Part model, mm, in its own coordinate system. A direction names the side the tool comes from. Round coordinates to 2 decimals unless told otherwise and drop trailing zeros. Loops run counter-clockwise (first coordinate to the right, second up) from the corner with the lowest first, then second, coordinate; pieces in that order, holes last. Notation, with made-up numbers: M -1.75,-11.5 L 57.25,-11.5 A19 cw 57.25,-7.5 Z; hole C 29,48 d9. An arc over 180 degrees is marked long. Answer as CSV lines item,"result". Start each with the question number.
Item 1: Band-saw the part on B-B (z = -5.5). Give the cut face in (x, y).
Item 2: Mould opens along Z. For faces 1 (the flat face through (123, 1.5, 0)), 2 (the flat face through (249, 1, 0)), 3 (the flat face through (123, 8, 20)) say: pulls with the +Z half, pulls with the -Z half, needs draft (parallel to the pull), parting line crosses it, or undercut.
Item 3: Which spindle directions (+Z, -Z, +X, -X, +Y, -Y) get a long thin tool onto all of the face, cutting with end or side? Do faces 4 (the flat face through (123, 8, -18.5)), 5 (the flat face through (123, 0, 0)). Say none if no direction does.
Item 4: Band-saw the part on A-A (x = 60.5). Give the cut face in (y, z), and give its area (4 significant figures).
Item 5: Drop flat-ended pins along their axis: pin 1 Ø2 at (x, y) = (91.67, 7.5) entering from +Z; pin 2 Ø11 at (x, z) = (143, 5) entering from +Y; pin 3 Ø8 at (y, z) = (4.5, -9) entering from +X. Give the stop position or say it passes through.
Item 6: Wall check: line 1 (Z direction, x = 132.5, y = 7.75); line 2 (Y direction, x = 25, z = 19); line 3 (Y direction, x = 109, z = -16.5). Give the ranges that are in metal, low to high.
```python
from build123d import *

# Parameters (mm, degrees)
SALIENTE_EXTRUIR1_DEPTH = 250
CROQUIS2_R              = 1.25
CORTAR_EXTRUIR1_DEPTH   = 41


with BuildPart() as part:
    # Croquis1 → Saliente-Extruir1 (new body)
    with BuildSketch(Plane(origin=(0, 0, 0), x_dir=(0, 0, -1), z_dir=(1, 0, 0))):
        Polygon((-20, 0), (20, 0), (20, 15), (18.5, 15), (18.5, 1.5), (-18.5, 1.5), (-18.5, 15), (-20, 15), align=None)
    extrude(amount=SALIENTE_EXTRUIR1_DEPTH)

    # Croquis2 → Cortar-Extruir1 (cut, through all)
    with BuildSketch(Plane(origin=(0, 0, -20), x_dir=(-1, 0, 0), z_dir=(0, 0, -1))):
        with Locations((-225, 7.5)):
            Circle(CROQUIS2_R)
        with Locations((-25, 7.5)):
            Circle(CROQUIS2_R)
        with Locations((-158.333333333, 7.5)):
            Circle(CROQUIS2_R)
        with Locations((-91.666666667, 7.5)):
            Circle(CROQUIS2_R)
        Polygon((0, 15), (-15, 15), (0, 0), align=None)
        Polygon((-250, 15), (-235, 15), (-250, 0), align=None)
    extrude(amount=-CORTAR_EXTRUIR1_DEPTH, mode=Mode.SUBTRACT)


solid = part.part
```
Answer block:
1,outline,"M 0,0 L 250,0 L 248.5,1.5 L 1.5,1.5 Z"
2,face 1,"undercut"
2,face 2,"needs draft"
2,face 3,"pulls with the +Z half"
3,face 4,"+X, -X, +Y"
3,face 5,"+Z, -Z, +X, -X, -Y"
4,outline,"M 0,-20 L 15,-20 L 15,-18.5 L 1.5,-18.5 L 1.5,18.5 L 15,18.5 L 15,20 L 0,20 Z"
4,area,"100.5 mm^2"
5,pin 1,"passes through"
5,pin 2,"stops at y = 1.5"
5,pin 3,"stops at x = 249.5"
6,line 1,"z = -20 to -18.5, 18.5 to 20"
6,line 2,"y = 0 to 6.25, 8.75 to 15"
6,line 3,"y = 0 to 1.5"
